```python
from build123d import *

# Parameters (mm, degrees)
SKETCH_2_R      = 2.025
SKETCH_2_R_2    = 3.1
EXTRUDE_1_DEPTH = 4
FILLET_1_R      = 5


with BuildPart() as part:
    # 草图2 → 凸台-拉伸1 (new body)
    with BuildSketch(Plane.XY):
        with BuildLine():
            Line((-22, 14.75), (-44.464667105, -30.539388734))
            ThreePointArc((-44.464667105, -30.539388734), (-43.214642655, -37.659851164), (-36.044914585, -38.586428599))
            Line((-36.044914585, -38.586428599), (7, -14.75))
            Line((7, -14.75), (7, 14.75))
            Line((7, 14.75), (-22, 14.75))
        make_face()
        with Locations((-4, 5)):
            Circle(SKETCH_2_R, mode=Mode.SUBTRACT)
        with Locations((-4, -5)):
            Circle(SKETCH_2_R, mode=Mode.SUBTRACT)
        with Locations((-39, -33.25)):
            Circle(SKETCH_2_R_2, mode=Mode.SUBTRACT)
    extrude(amount=EXTRUDE_1_DEPTH)

    # 圆角1
    fillet_1_edges = [part.edges().sort_by_distance(p)[0] for p in [
        (-22, 14.75, 2),
        (7, 14.75, 2),
        (7, -14.75, 2),
    ]]
    fillet(fillet_1_edges, radius=FILLET_1_R)


solid = part.part
```
The model under review builds one solid part; all positions refer to its coordinate system, in mm. Round coordinates to 2 decimals unless told otherwise and drop trailing zeros. Write each loop counter-clockwise with the first axis right and the second up, starting at its lowest first coordinate (ties: lowest second). Pieces come first, ordered by that corner, then holes.
(1) Wall thickness on L1, parallel to Y at x = -3, z = 3.75; L2, parallel to Y at x = -4, z = 1.05 (3 decimals); L3, parallel to X at y = 6, z = 0.9: over which ranges is each line inside the solid? List them lowest first.
(2) We need section A-A on z = 1.35. Give the boundary of the cut face in (x, y) (3 decimals), and give its area (3 significant figures).
(3) We need section D-D on x = -39. Give the boundary of the cut face in (y, z), and give its area (3 significant figures).
(4) Insertion check: pin 1 (3 mm diameter, centred on x = -4, y = -5, fed in from -Z). The pin has a flat end and moves straight along its axis. Give the tip position at first contact, or say it passes through.
(5) We need section C-C on x = -4. Give the boundary of the cut face in (y, z) (3 decimals).
(6) Mouldability with a two-part tool opening along Y and no side actions: class faces 1 (the cylindrical face through (-5.61, 3.77, 1.97)), 2 (the cylindrical face through (-43.292, -37.584, 1.972)), 3 (the cylindrical face through (-21.567, 13.978, 2.028)) as +Y half, -Y half, draft (parallel to the pull), parting line (faces both ways), or undercut.
(7) We need section B-B on y = -5. Give the boundary of the cut face in (x, z) (1 decimal), and give its area (3 significant figures).
Findings below:
1. L1: y = -20.29 to -6.76, -3.24 to 3.24, 6.76 to 14.75
1. L2: y = -20.841 to -7.025, -2.975 to 2.975, 7.025 to 14.75
1. L3: x = -26.34 to -5.76, -2.24 to 7
2. outline: (-44.465, -30.539) arc R6.1 ccw to (-36.045, -38.586) - (4.422, -16.177) arc R5 ccw to (7, -11.803) - (7, 9.75) arc R5 ccw to (2, 14.75) - (-18.899, 14.75) arc R5 ccw to (-23.378, 11.972) - close; hole circle Ø6.2 at (-39, -33.25); hole circle Ø4.05 at (-4, -5); hole circle Ø4.05 at (-4, 5)
2. area: 1,660 mm2
3. outline: (-39.35, 0) - (-36.35, 0) - (-36.35, 4) - (-39.35, 4) - close; (-30.15, 0) - (-19.52, 0) - (-19.52, 4) - (-30.15, 4) - close
3. area: 54.5 mm2
4. pin 1: passes through
5. outline: (-20.841, 0) - (-7.025, 0) - (-7.025, 4) - (-20.841, 4) - close; (-2.975, 0) - (2.975, 0) - (2.975, 4) - (-2.975, 4) - close; (7.025, 0) - (14.75, 0) - (14.75, 4) - (7.025, 4) - close
6. face 1: undercut
6. face 2: parting line
6. face 3: +Y half
7. outline: (-31.8, 0) - (-6, 0) - (-6, 4) - (-31.8, 4) - close; (-2, 0) - (7, 0) - (7, 4) - (-2, 4) - close
7. area: 139 mm2
